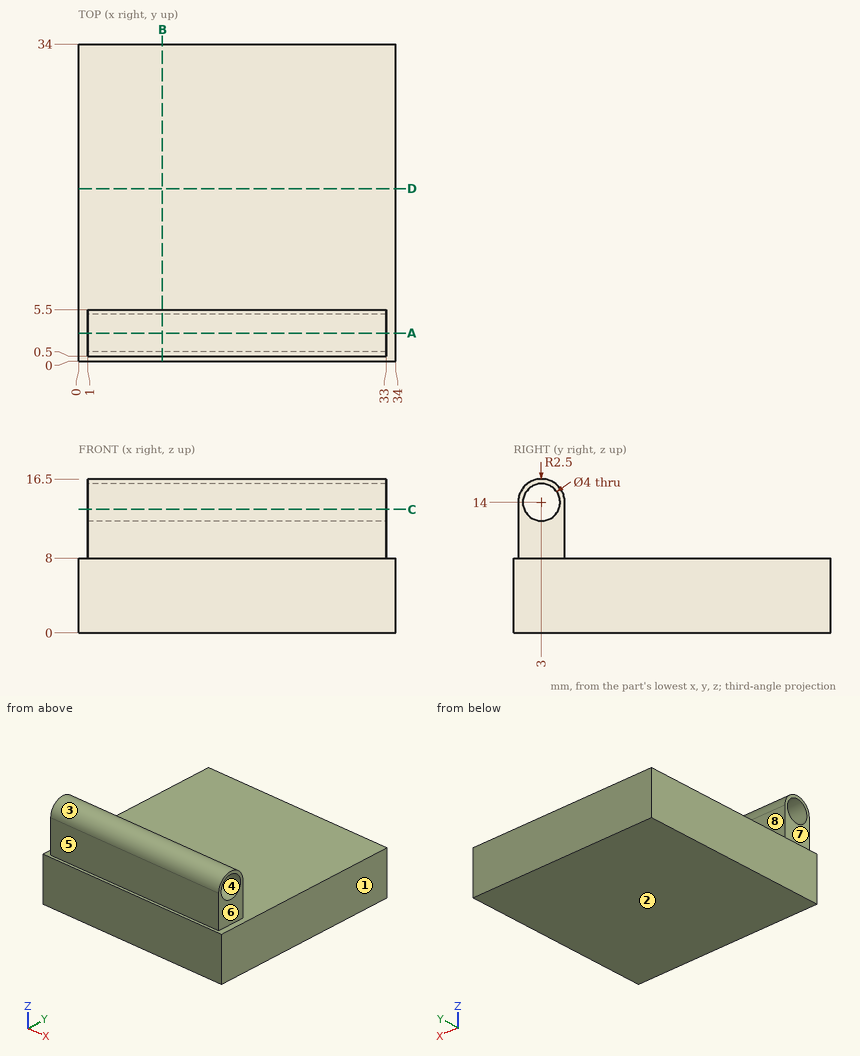
Source: three-view drawing plus pictorial views. Frame: mm from the lowest corner of the part. A direction names the side the tool comes from. Give positions to 0.01 mm unless a question says otherwise; leave off trailing zeros. Write each loop counter-clockwise with the first axis right and the second up, starting at its lowest first coordinate (ties: lowest second). Pieces come first, ordered by that corner, then holes. Notation, with made-up numbers: (17.5, 30.5) -> (60.5, 30.5) arc R20 ccw to (60.5, 56.5) -> close; hole circle Ø3 at (19, 24). An arc over 180 degrees is marked (long way). Answer in a Markdown table with one row per item.
(1) Pin query (flat end, axial travel): pin 1 (8 mm diameter, centred on x = 13, z = 14, fed in from -Y); pin 2 (5 mm diameter, centred on y = 3, z = 14, fed in from -X); pin 3 (1.5 mm diameter, centred on y = 3.5, z = 10.5, fed in from +X). Return the tip coordinate at first contact, or that it passes through.
Answers below:
| item | result |
|---|---|
| pin 1 | y = 0.5 |
| pin 2 | x = 1 |
| pin 3 | x = 33 |
(2) Section query A-A on y = 3. Return loops of the section in (x, z), then the cut area to 3 significant figures.
Answers below:
| item | result |
|---|---|
| outline | (0, 0) -> (34, 0) -> (34, 8) -> (33, 8) -> (33, 12) -> (1, 12) -> (1, 8) -> (0, 8) -> close; (1, 16) -> (33, 16) -> (33, 16.5) -> (1, 16.5) -> close |
| area | 416 mm^2 |
(3) Ray query, line 1 along Y through (x, z) = (9, 14); line 2 along Z through (x, y) = (30.5, 15); line 3 along X through (y, z) = (2, 12). Return the intervals inside material, ascending. Write a range as [from, to].
Answers below:
| item | result |
|---|---|
| line 1 | [0.5, 1], [5, 5.5] |
| line 2 | [0, 8] |
| line 3 | [1, 33] |
(4) Set-up query: the marked faces 5, 6, 7 and 8. Return all of +Z, -Z, +X, -X, +Y, -Y with unobstructed straight access to the full face (end or side cutting, diameter ignored); none if empty.
Answers below:
| item | result |
|---|---|
| face 5 | +Z, +X, -X, -Y |
| face 6 | +Z, +X, +Y, -Y |
| face 7 | +Z, -X, +Y, -Y |
| face 8 | +Z, +X, -X, +Y |
(5) Section query B-B on x = 9. Return loops of the section in (y, z), then the cut area to 3 significant figures.
Answers below:
| item | result |
|---|---|
| outline | (0, 0) -> (34, 0) -> (34, 8) -> (5.5, 8) -> (5.5, 14) arc R2.5 ccw to (0.5, 14) -> (0.5, 8) -> (0, 8) -> close; hole circle Ø4 at (3, 14) |
| area | 299 mm^2 |
(6) Section query D-D on y = 18.5. Return loops of the section in (x, z), then the cut area to 3 significant figures.
Answers below:
| item | result |
|---|---|
| outline | (0, 0) -> (34, 0) -> (34, 8) -> (0, 8) -> close |
| area | 272 mm^2 |
(7) Section query C-C on z = 13.25. Return loops of the section in (x, y).
Answers below:
| item | result |
|---|---|
| outline | (1, 0.5) -> (33, 0.5) -> (33, 1.15) -> (1, 1.15) -> close; (1, 4.85) -> (33, 4.85) -> (33, 5.5) -> (1, 5.5) -> close |
(8) Draft query along Z for the marked faces 1, 2, 3 and 4. Return one class per face: +Z half, -Z half, draft (parallel to the pull), parting line (faces both ways), or undercut.
Answers below:
| item | result |
|---|---|
| face 1 | draft |
| face 2 | -Z half |
| face 3 | +Z half |
| face 4 | undercut |
